Design review of the part built by this model. Coordinates are the model's own, in mm. Coordinates: 2 decimals unless noted, no trailing zeros. Write each loop counter-clockwise with the first axis right and the second up, starting at its lowest first coordinate (ties: lowest second). Pieces come first, ordered by that corner, then holes. Notation, with made-up numbers: M -15,-17 L 44,-17 A12 ccw 44,5 Z; hole C 89.5,85 d6. An arc over 180 degrees is marked long. Return JSON: item names as keys, results as strings. Group by question number.
```python
from build123d import *
from OCP.BRepFilletAPI import BRepFilletAPI_MakeChamfer

# Parameters (mm, degrees)
BOSS_EXTRUDE1_DEPTH = 20
FILLET1_R           = 10
CHAMFER1_SIZE       = 3
CHAMFER1_SIZE2      = 5.019471555
SKETCH5_R           = 5
FILLET4_R           = 10
FILLET5_R           = 0.5


with BuildPart() as part:
    # Sketch1 → Boss-Extrude1 (new body)
    with BuildSketch(Plane(origin=(0, 0, 0), x_dir=(0, 0, -1), z_dir=(1, 0, 0))):
        with BuildLine():
            Line((-86, 0), (-67, 0))
            Line((-67, 0), (-67, 1))
            Line((-67, 1), (-19, 1))
            Line((-19, 1), (-19, 0))
            Line((-19, 0), (0, 0))
            Line((0, 0), (0, 10))
            Line((0, 10), (-11.889492676, 14.327421434))
            ThreePointArc((-11.889492676, 14.327421434), (-43, 38.835002999), (-74.110507324, 14.327421434))
            Line((-74.110507324, 14.327421434), (-86, 10))
            Line((-86, 10), (-86, 0))
        make_face()
    extrude(amount=BOSS_EXTRUDE1_DEPTH)

    # Fillet1
    fillet1_edges = [part.edges().sort_by_distance(p)[0] for p in [
        (10, 14.327421434, 74.110507324),
        (10, 14.327421434, 11.889492676),
    ]]
    fillet(fillet1_edges, radius=FILLET1_R)

    # Chamfer1: one chamfer whose edges measure the first distance from different faces: ONE call of the kernel's chamfer builder (chamfer() names one face for all edges)
    chamfer1_edges_1 = [part.edges().sort_by_distance(p)[0] for p in [
        (10, 10, 86),
    ]]
    chamfer1_side_1 = [part.faces().sort_by_distance(p)[0] for p in [
        (10, 11.323089013, 82.364842814),
    ]]
    chamfer1_edges_2 = [part.edges().sort_by_distance(p)[0] for p in [
        (10, 10, 0),
    ]]
    chamfer1_side_2 = [part.faces().sort_by_distance(p)[0] for p in [
        (10, 5, 0),
    ]]
    chamfer1 = BRepFilletAPI_MakeChamfer(part.part.solid().wrapped)
    for e in chamfer1_edges_1:
        chamfer1.Add(CHAMFER1_SIZE, CHAMFER1_SIZE2, e.wrapped, chamfer1_side_1[0].wrapped)  # the first distance lies on this face
    for e in chamfer1_edges_2:
        chamfer1.Add(CHAMFER1_SIZE, CHAMFER1_SIZE2, e.wrapped, chamfer1_side_2[0].wrapped)  # the first distance lies on this face
    add(Compound.cast(chamfer1.Shape()), mode=Mode.REPLACE)

    # augu cut: sweep along a path in Sketch2
    with BuildLine(Plane(origin=(10, 0, 0), x_dir=(0, 0, -1), z_dir=(1, 0, 0))) as augu_cut_path:
        Line((-10.5, -11.403017839), (-10.5, 10))
        ThreePointArc((-10.5, 10), (-43, 42.5), (-75.5, 10))
        Line((-75.5, 10), (-75.5, -11.403017839))
    # Sketch5 → augu cut (sweep, cut)
    with BuildSketch(Plane(origin=(0, -11.403017839, 0), x_dir=(-1, 0, 0), z_dir=(0, -1, 0))):
        with Locations((-10, -10.5)):
            Circle(SKETCH5_R)
    sweep(path=augu_cut_path.line, mode=Mode.SUBTRACT)

    # Sketch6 → Cut-Revolve2 (revolve, cut)
    with BuildSketch(Plane.XZ.offset(1)):
        with BuildLine():
            Line((0, 64), (1.5, 64))
            Line((1.5, 64), (1.5, 64.9089023))
            ThreePointArc((1.5, 64.9089023), (10, 66.5), (18.5, 64.9089023))
            Line((18.5, 64.9089023), (18.5, 64))
            Line((18.5, 64), (20, 64))
            Line((20, 64), (20, 43))
            Line((20, 43), (0, 43))
            Line((0, 43), (0, 64))
        make_face()
    revolve(axis=Axis((0, -1, 43), (1, 0, 0)), mode=Mode.SUBTRACT)

    # Fillet4
    fillet4_edges = [part.edges().sort_by_distance(p)[0] for p in [
        (10, 7, 0),
        (10, 4.980528445, 86),
    ]]
    fillet(fillet4_edges, radius=FILLET4_R)

    # Fillet5
    fillet5_edges = [part.edges().sort_by_distance(p)[0] for p in [
        (1.5, 20.9089023, 43),
        (18.5, 20.9089023, 43),
        (18.5, 20, 43),
        (1.5, 20, 43),
    ]]
    fillet(fillet5_edges, radius=FILLET5_R)


solid = part.part
```
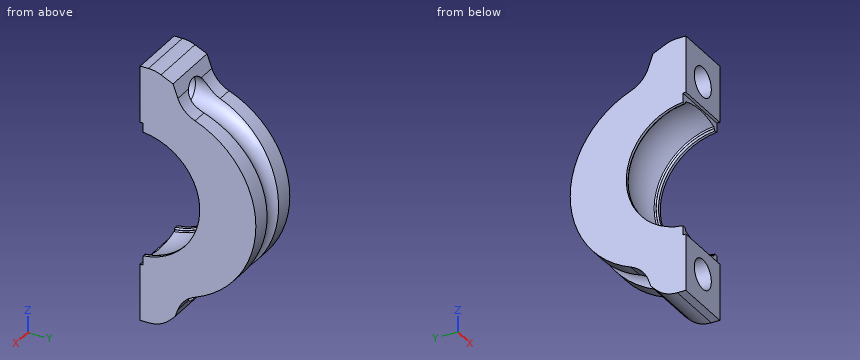
Item 1: For line 1 (Z direction, x = 10, y = 7); line 2 (Z direction, x = 10, y = 2.25); line 3 (X direction, y = 4.25, z = 75.5), list the stretches that pass through material, from the lowest coordinate up.
Item 2: For pin 1 (21.5 mm diameter, centred on y = 15.5, z = 47, fed in from +X); pin 2 (1.5 mm diameter, centred on x = 7.5, z = 63, fed in from +Y); pin 3 (5 mm diameter, centred on x = 3.5, z = 44, fed in from -Y); pin 4 (1 mm diameter, centred on x = 11.5, z = 47.5, fed in from +Y), all flat-tipped, find the tip position at first contact; note any pin that passes through.
Item 3: Add section A-A (x = 10). Write out the cut boundary in (y, z), plus the area to 3 significant figures.
Geometry check:
{
 "1": {"line 1": "0.9 to 5.5, 15.5 to 20.9, 65.1 to 70.5, 80.5 to 85.06", "line 2": "0 to 5.5, 15.5 to 19.73, 66.27 to 70.5, 80.5 to 86", "line 3": "0 to 5, 15 to 20"},
 "2": {"pin 1": "x = 20", "pin 2": "y = 30.85", "pin 3": "y = 19.94", "pin 4": "y = 37.57"},
 "3": {"outline": "M 0,0 L 2.86,0 A10 ccw 9.93,2.93 L 11.72,4.72 L 12.02,5.55 A37.5 cw 10,5.5 L 0,5.5 Z; M 0,15.5 L 10,15.5 A27.5 ccw 10,70.5 L 0,70.5 L 0,67 L 1,67 L 1,66.41 A23.5 cw 1,19.59 L 1,19 L 0,19 Z; M 0,80.5 L 10,80.5 A37.5 cw 12.02,80.45 L 11.03,83.18 L 6.99,85.06 A10 ccw 2.76,86 L 0,86 Z", "area": "1,020 mm^2"}
}
